Model file for the job. Use its own axes, mm. Face numbers are marked on the shaded views. Round coordinates to 2 decimals unless told otherwise and drop trailing zeros. Loops run counter-clockwise (first coordinate to the right, second up) from the corner with the lowest first, then second, coordinate; pieces in that order, holes last. Notation, with made-up numbers: M -6.5,-1 L 32.5,-1 A9 ccw 32.5,7 Z; hole C 69,73.5 d1. An arc over 180 degrees is marked long. Use a Markdown table: item, result. Add a question column.
Item 1: Saw through at B-B on y = -7.84. Write the cut outline in (x, z), then the cut area to 3 significant figures.
Item 2: Wall check: L1, parallel to Y at x = 9.85, z = -93.5; L2, parallel to Y at x = 3.75, z = -19; L3, parallel to Z at x = 1.75, y = 5. Give the ranges that are in metal, low to high. Write a range as from..to.
Item 3: Pin check, flat tips, straight feed: P1, Ø0.8, axis at x = 9.5, z = 6, coming from the +Y side; P2, Ø1, axis at x = 6.5, z = -72.5, coming from the +Y side; P3, Ø2.5, axis at x = 7, y = -14.5, coming from the -Z side; P4, Ø10, axis at y = -6.5, z = -91, coming from the -X side. Stop position of each tip, or through.
Item 4: Saw through at A-A on z = -112.5. Write the cut outline in (x, y).
Item 5: Saw through at C-C on x = 7.25. Write the cut outline in (y, z).
Item 6: Two-plate mould, pull along Z, no slides. Class the marked faces 1, 2 and 3: +Z half, -Z half, draft (parallel to the pull), parting line (faces both ways), or undercut.
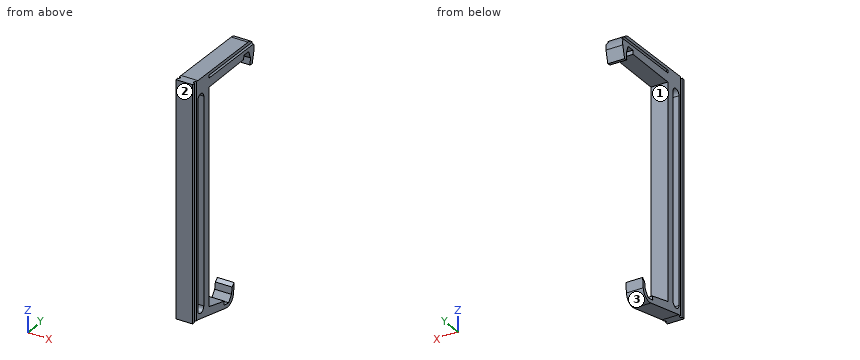
```python
from build123d import *

# Parameters (mm, degrees)
BOSS_EXTRUDE1_DEPTH = 10
CUT_EXTRUDE4_REACH  = 150.602
CUT_EXTRUDE5_DEPTH  = 144.972857609


with BuildPart() as part:
    # Sketch1 → Boss-Extrude1 (new body)
    with BuildSketch(Plane(origin=(0, 0, 0), x_dir=(0, 0, -1), z_dir=(1, 0, 0))):
        with BuildLine():
            Line((0, 0), (128, 0))
            Line((128, 0), (131.946990438, 14.730368851))
            Line((131.946990438, 14.730368851), (134.217403847, 14.362642119))
            Line((134.217403847, 14.362642119), (134.952857311, 18.903468939))
            Line((134.952857311, 18.903468939), (131.341565092, 21.580990302))
            Line((131.341565092, 21.580990302), (127.393020031, 22.220515053))
            Line((127.393020031, 22.220515053), (125.710603817, 24.179837998))
            Line((125.710603817, 24.179837998), (131.520951621, 23.60910455))
            ThreePointArc((131.520951621, 23.60910455), (135.810577018, 21.133985308), (136.778030397, 16.276914661))
            Line((136.778030397, 16.276914661), (130.5, -10.68))
            Line((130.5, -10.68), (130.5, -15.68))
            Line((130.5, -15.68), (-9, -15.68))
            Line((-9, -15.68), (-9, -10.68))
            Line((-9, -10.68), (-8.008635101, 37.449655704))
            ThreePointArc((-8.008635101, 37.449655704), (-5.691899097, 42.063492927), (-0.648979735, 43.169713494))
            Line((-0.648979735, 43.169713494), (6.548278337, 41.493534839))
            Line((6.548278337, 41.493534839), (6.242876448, 39.365871735))
            Line((6.242876448, 39.365871735), (2.263353613, 39.770096924))
            Line((2.263353613, 39.770096924), (-2.28822563, 38.082429484))
            Line((-2.28822563, 38.082429484), (-2.28822563, 33.482429484))
            Line((-2.28822563, 33.482429484), (0, 33.25))
            Line((0, 33.25), (0, 0))
        make_face()
        with BuildLine():
            Line((2.84, -5), (125.16, -5))
            ThreePointArc((125.16, -5), (128, -7.84), (125.16, -10.68))
            Line((125.16, -10.68), (2.84, -10.68))
            ThreePointArc((2.84, -10.68), (0, -7.84), (2.84, -5))
        make_face(mode=Mode.SUBTRACT)
    extrude(amount=BOSS_EXTRUDE1_DEPTH)

    # Cut-Extrude4: up to this plane
    cut_extrude4_end = Plane(origin=(0, 0, 0), z_dir=(0, 1, 0))
    # Sketch2 → Cut-Extrude4 (cut, up to the surface)
    with BuildSketch(Plane(origin=(0, 43.267611016, -0.891217487), x_dir=(1, 0, 0), z_dir=(0, 0.9997879328481811, -0.020593429320073266)), mode=Mode.PRIVATE) as cut_extrude4_sk1:
        with BuildLine():
            Line((0, -5.291493544), (0, -6.964813597))
            ThreePointArc((0, -6.964813597), (1, -6.12815357), (0, -5.291493544))
        make_face()
    cut_extrude4_tool1 = split(extrude(cut_extrude4_sk1.sketch, amount=-CUT_EXTRUDE4_REACH, mode=Mode.PRIVATE), bisect_by=cut_extrude4_end, keep=Keep.BOTH, mode=Mode.PRIVATE)
    cut_extrude4 = cut_extrude4_tool1.solids().sort_by_distance((0.431182, 43.393811, 5.235637))[0]
    add(cut_extrude4, mode=Mode.SUBTRACT)

    # Mirror1: Cut-Extrude4 across plane
    add(cut_extrude4.mirror(Plane(origin=(5, 0, 0), x_dir=(0, 0, 1), z_dir=(1, 0, 0))), mode=Mode.SUBTRACT)

    # Sketch3 → Cut-Extrude5 (cut, symmetric)
    with BuildSketch(Plane.XY):
        with BuildLine():
            ThreePointArc((0, -13.866660027), (1, -13.03), (0, -12.193339973))
            Line((0, -12.193339973), (0, -13.866660027))
        make_face()
    cut_extrude5 = extrude(amount=CUT_EXTRUDE5_DEPTH, both=True, mode=Mode.SUBTRACT)

    # Mirror2: Cut-Extrude5 across plane
    add(cut_extrude5.mirror(Plane(origin=(5, 0, 0), x_dir=(0, 0, 1), z_dir=(1, 0, 0))), mode=Mode.SUBTRACT)


solid = part.part
```
Entries:
| question | item | result |
|---|---|---|
| 1 | outline | M 0,-131.16 L 10,-131.16 L 10,-128 L 0,-128 Z; M 0,0 L 10,0 L 10,8.94 L 0,8.94 Z |
| 1 | area | 121 mm2 |
| 2 | L1 | -15.68..-13.88, -12.18..-10.68, -5..0 |
| 2 | L2 | -15.68..-10.68, -5..0 |
| 2 | L3 | -134.15..-129.34, 0..8.68 |
| 3 | P1 | y = 42 |
| 3 | P2 | y = 0 |
| 3 | P3 | z = -130.5 |
| 3 | P4 | x = 0 |
| 4 | outline | M 0,-15.68 L 10,-15.68 L 10,-13.87 A0.85 cw long 10,-12.19 L 10,-10.68 L 0,-10.68 L 0,-12.19 A0.85 cw long 0,-13.87 Z; M 0,-5 L 10,-5 L 10,0 L 0,0 Z |
| 5 | outline | M -15.68,-130.5 L -10.68,-130.5 L 16.28,-136.78 A6 ccw 23.61,-131.52 L 24.18,-125.71 L 22.22,-127.39 L 21.58,-131.34 L 18.9,-134.95 L 14.36,-134.22 L 14.73,-131.95 L 0,-128 L 0,0 L 33.25,0 L 33.48,2.29 L 38.08,2.29 L 39.77,-2.26 L 39.37,-6.24 L 41.49,-6.55 L 43.17,0.65 A6 ccw 37.45,8.01 L -10.68,9 L -15.68,9 Z; hole M -10.68,-125.16 A2.84 ccw -5,-125.16 L -5,-2.84 A2.84 ccw -10.68,-2.84 Z |
| 6 | face 1 | undercut |
| 6 | face 2 | draft |
| 6 | face 3 | -Z half |
